Could you check a few things on this model? Use its own coordinates, in mm. Face numbers are marked on the shaded views. A direction names the side the tool comes from. Coordinates: 2 decimals unless noted, no trailing zeros. Write each loop counter-clockwise with the first axis right and the second up, starting at its lowest first coordinate (ties: lowest second). Pieces come first, ordered by that corner, then holes. Notation, with made-up numbers: (80.25, 9.5) - (122.25, 9.5) arc R24 ccw to (122.25, 23.5) - close; hole circle Ø11 at (-6, 68.25). An arc over 180 degrees is marked (long way). Answer as a JSON object with one key per item and string values. Group by question number.
1) Please list where these lines run through material, in increasing order: line 1 along Y through (x, z) = (0, 6); line 2 along Y through (x, z) = (-1, 8.5); line 3 along Z through (x, y) = (18, 7).
2) If we section it at B-B (z = 25): Write out the boundary of the cut face in (x, y), plus the area to 3 significant figures.
3) We'd pull the mould along X, two halves only. Please class the marked faces 4, 5 and 6: released by +X, released by -X, zero draft, split by the parting line, or undercut.
4) If we section it at A-A (z = 32): Write out the boundary of the cut face in (x, y).
5) Will these pins go through, and if not, where does the flat tip stop? pin 1 Ø8 at (x, y) = (11, 9.5) entering from +Z; pin 2 Ø6 at (x, y) = (-1, 3.5) entering from -Z; pin 3 Ø1 at (x, z) = (1, 10) entering from +Y.
6) On a 3-axis mill with a long thin cutter (end or side, diameter ignored), from which of +Z, -Z, +X, -X, +Y, -Y can I reach the whole of each face in a straight line? I mean the marked faces 1, 2 and 3. Say none if no direction works.
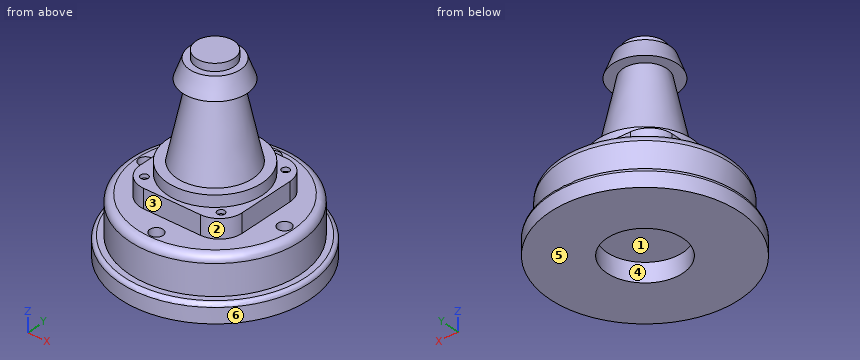
```python
from build123d import *

# Parameters (mm, degrees)
SKETCH1_R             = 25
BOSS_EXTRUDE1_DEPTH   = 5
SKETCH2_R             = 22.5
BOSS_EXTRUDE2_DEPTH   = 10
SKETCH3_W             = 27
SKETCH3_H             = 27
BOSS_EXTRUDE3_DEPTH   = 5
SKETCH5_R             = 12.5
BOSS_EXTRUDE4_DEPTH   = 3
SKETCH6_R             = 10
BOSS_EXTRUDE5_DEPTH   = 20
BOSS_EXTRUDE5_TAPER   = 12
SKETCH7_R             = 8.5
BOSS_EXTRUDE6_DEPTH   = 5
BOSS_EXTRUDE6_TAPER   = 20
SKETCH8_R             = 5
BOSS_EXTRUDE7_DEPTH   = 2
FILLET1_R             = 6
SKETCH10_R            = 1.75
CUT_EXTRUDE2_DEPTH    = 5
SKETCH11_R            = 1
CUT_EXTRUDE3_DEPTH    = 1
SKETCH12_R            = 10
CUT_EXTRUDE4_DEPTH    = 5
FILLET2_R             = 2
FILLET3_R             = 1
BODY_MOVE_COPY2_ANGLE = 90


with BuildPart() as part:
    # Sketch1 → Boss-Extrude1 (new body)
    with BuildSketch(Plane(origin=(0, 0, 0), x_dir=(1, 0, 0), z_dir=(0, 1, 0))):
        Circle(SKETCH1_R)
    extrude(amount=BOSS_EXTRUDE1_DEPTH)

    # Sketch2 → Boss-Extrude2 (add)
    with BuildSketch(Plane(origin=(0, 5, 0), x_dir=(1, 0, 0), z_dir=(0, 1, 0))):
        Circle(SKETCH2_R)
    extrude(amount=BOSS_EXTRUDE2_DEPTH)

    # Sketch3 → Boss-Extrude3 (add)
    with BuildSketch(Plane(origin=(0, 15, 0), x_dir=(1, 0, 0), z_dir=(0, 1, 0))):
        Rectangle(SKETCH3_W, SKETCH3_H)
    extrude(amount=BOSS_EXTRUDE3_DEPTH)

    # Sketch5 → Boss-Extrude4 (add)
    with BuildSketch(Plane(origin=(0, 20, 0), x_dir=(1, 0, 0), z_dir=(0, 1, 0))):
        Circle(SKETCH5_R)
    extrude(amount=BOSS_EXTRUDE4_DEPTH)

    # Sketch6 → Boss-Extrude5 (add)
    with BuildSketch(Plane(origin=(0, 23, 0), x_dir=(1, 0, 0), z_dir=(0, 1, 0))):
        Circle(SKETCH6_R)
    extrude(amount=BOSS_EXTRUDE5_DEPTH, taper=BOSS_EXTRUDE5_TAPER)

    # Sketch7 → Boss-Extrude6 (add)
    with BuildSketch(Plane(origin=(0, 43, 0), x_dir=(1, 0, 0), z_dir=(0, 1, 0))):
        Circle(SKETCH7_R)
    extrude(amount=BOSS_EXTRUDE6_DEPTH, taper=BOSS_EXTRUDE6_TAPER)

    # Sketch8 → Boss-Extrude7 (add)
    with BuildSketch(Plane(origin=(0, 48, 0), x_dir=(1, 0, 0), z_dir=(0, 1, 0))):
        Circle(SKETCH8_R)
    extrude(amount=BOSS_EXTRUDE7_DEPTH)

    # Fillet1
    fillet1_edges = [part.edges().sort_by_distance(p)[0] for p in [
        (13.5, 17.5, 13.5),
        (13.5, 17.5, -13.5),
        (-13.5, 17.5, -13.5),
        (-13.5, 17.5, 13.5),
    ]]
    fillet(fillet1_edges, radius=FILLET1_R)

    # Sketch10 → Cut-Extrude2 (cut)
    with BuildSketch(Plane(origin=(0, 15, 0), x_dir=(1, 0, 0), z_dir=(0, 1, 0))):
        with Locations((-18.379384185, 0)):
            Circle(SKETCH10_R)
        with Locations((0, 18.400220003)):
            Circle(SKETCH10_R)
    cut_extrude2 = extrude(amount=-CUT_EXTRUDE2_DEPTH, mode=Mode.SUBTRACT)

    # Sketch11 → Cut-Extrude3 (cut)
    with BuildSketch(Plane(origin=(0, 20, 0), x_dir=(1, 0, 0), z_dir=(0, 1, 0))):
        with Locations((10.139251665, 10.139251665)):
            Circle(SKETCH11_R)
        with Locations((-10.139251665, 10.139251665)):
            Circle(SKETCH11_R)
    cut_extrude3 = extrude(amount=-CUT_EXTRUDE3_DEPTH, mode=Mode.SUBTRACT)

    # Mirror4: Cut-Extrude2, Cut-Extrude3 across plane
    add(cut_extrude2.mirror(Plane.XY), mode=Mode.SUBTRACT)
    add(cut_extrude3.mirror(Plane.XY), mode=Mode.SUBTRACT)

    # Mirror6: Cut-Extrude2 across plane
    add(cut_extrude2.mirror(Plane(origin=(0, 0, 0), x_dir=(0, 0, 1), z_dir=(1, 0, 0))), mode=Mode.SUBTRACT)

    # Sketch12 → Cut-Extrude4 (cut)
    with BuildSketch(Plane.XZ):
        Circle(SKETCH12_R)
    extrude(amount=-CUT_EXTRUDE4_DEPTH, mode=Mode.SUBTRACT)

    # Fillet2
    fillet2_edges = [part.edges().sort_by_distance(p)[0] for p in [
        (-22.5, 15, 0),
    ]]
    fillet(fillet2_edges, radius=FILLET2_R)

    # Fillet3
    fillet3_edges = [part.edges().sort_by_distance(p)[0] for p in [
        (-25, 5, 0),
    ]]
    fillet(fillet3_edges, radius=FILLET3_R)


with BuildPart() as part_1:
    # Body-Move/Copy1: moved
    add(part.part.moved(Location((0, -5, 0))))


with BuildPart() as part_2:
    # Body-Move/Copy2: moved
    add(part_1.part.rotate(Axis((0, 0, 0), (1, 0, 0)), BODY_MOVE_COPY2_ANGLE))


solid = part_2.part
```
Here are the results:
{
 "1": {"line 1": "y = -22.5 to -20.15, -16.65 to 16.65, 20.15 to 22.5", "line 2": "y = -22.41 to -19.84, -16.96 to 16.96, 19.84 to 22.41", "line 3": "z = -5 to 10"},
 "2": {"outline": "circle Ø17.02 at (0, 0)", "area": "228 mm²"},
 "3": {"face 4": "undercut", "face 5": "zero draft", "face 6": "split by the parting line"},
 "4": {"outline": "circle Ø14.05 at (0, 0)"},
 "5": {"pin 1": "stops at z = 18", "pin 2": "stops at z = 0", "pin 3": "stops at y = 21.8"},
 "6": {"face 1": "-Z", "face 2": "+Z, +X, -Y", "face 3": "+Z, +X, -X, -Y"}
}
